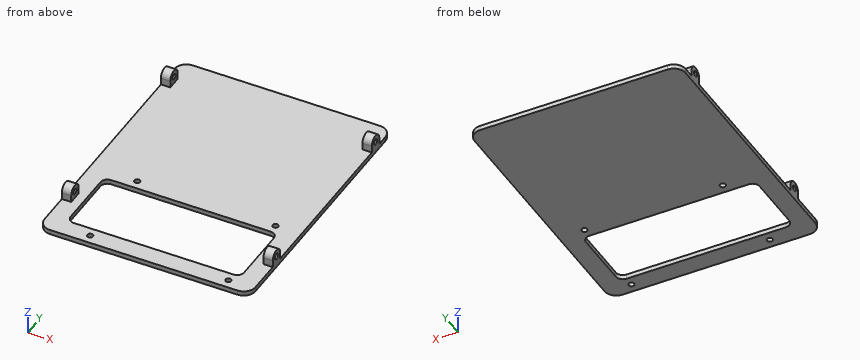
```python
from build123d import *

# Parameters (mm, degrees)
SKETCH1_R                        = 1.524
SCREW_HOLES_DEPTH                = 5.08
SCREW_HOLES_2_DEPTH              = 5.08
SKETCH2_W                        = 2.54
SKETCH2_H                        = 146.05
MAIN_EXTRUDE_DEPTH               = 114.3
FILLET1_R                        = 6.35
SKETCH3_R                        = 1.524
COMPONENT_MOUNT_HOLES_DEPTH      = 8.62
COMPONENT_MOUNT_HOLES_DEPTH_BACK = 3.54
SKETCH4_W                        = 93.98
SKETCH4_H                        = 38.1
WEIGHT_REDUCTION_DEPTH           = 8.62
WEIGHT_REDUCTION_DEPTH_BACK      = 3.54
FILLET2_R                        = 3.81


with BuildPart() as part:
    # Sketch1 → Screw holes (new body)
    with BuildSketch(Plane(origin=(0, 0, 0), x_dir=(0, 0, -1), z_dir=(1, 0, 0))):
        with BuildLine():
            Line((0, 46.99), (3.81, 46.99))
            Line((3.81, 46.99), (3.81, 54.61))
            Line((3.81, 54.61), (0, 54.61))
            ThreePointArc((0, 54.61), (-3.81, 50.8), (0, 46.99))
        make_face()
        with Locations((0, 50.8)):
            Circle(SKETCH1_R, mode=Mode.SUBTRACT)
    screw_holes = extrude(amount=SCREW_HOLES_DEPTH)



with BuildPart() as body_2:
    # Sketch1 → Screw holes 2 (new body)
    with BuildSketch(Plane(origin=(0, 0, 0), x_dir=(0, 0, -1), z_dir=(1, 0, 0))):
        with BuildLine():
            Line((3.81, -54.61), (0, -54.61))
            ThreePointArc((0, -54.61), (-3.81, -50.8), (0, -46.99))
            Line((0, -46.99), (3.81, -46.99))
            Line((3.81, -46.99), (3.81, -54.61))
        make_face()
        with Locations((0, -50.8)):
            Circle(SKETCH1_R, mode=Mode.SUBTRACT)
    screw_holes_2 = extrude(amount=SCREW_HOLES_2_DEPTH)


with BuildPart() as part_1:
    add(part.part)

    add(body_2.part)  # Main extrude merges body 2
    # Sketch2 → Main extrude (add)
    with BuildSketch(Plane.ZY):
        with Locations((-5.08, -5.715)):
            Rectangle(SKETCH2_W, SKETCH2_H)
    extrude(amount=-MAIN_EXTRUDE_DEPTH)

    # Screw holes 2 2: Screw holes, Screw holes 2 across plane
    add(screw_holes.mirror(Plane.ZY.offset(-57.15)))
    add(screw_holes_2.mirror(Plane.ZY.offset(-57.15)))

    # Fillet1
    fillet1_edges = [part_1.edges().sort_by_distance(p)[0] for p in [
        (114.3, -78.74, -5.08),
        (114.3, 67.31, -5.08),
        (0, 67.31, -5.08),
        (0, -78.74, -5.08),
    ]]
    fillet(fillet1_edges, radius=FILLET1_R)

    # Sketch3 → Component mount holes (cut, two sides)
    with BuildSketch(Plane.XY.offset(-3.81)) as component_mount_holes_sk:
        with Locations((25.4, -25.4)):
            Circle(SKETCH3_R)
        with Locations((100.33, -25.4)):
            Circle(SKETCH3_R)
        with Locations((100.33, -73.66)):
            Circle(SKETCH3_R)
        with Locations((25.4, -73.66)):
            Circle(SKETCH3_R)
    extrude(amount=COMPONENT_MOUNT_HOLES_DEPTH, mode=Mode.SUBTRACT)
    extrude(component_mount_holes_sk.sketch, amount=-COMPONENT_MOUNT_HOLES_DEPTH_BACK, mode=Mode.SUBTRACT)

    # Sketch4 → Weight reduction (cut, two sides)
    with BuildSketch(Plane.XY.offset(-3.81)) as weight_reduction_sk:
        with Locations((57.15, -49.53)):
            Rectangle(SKETCH4_W, SKETCH4_H)
    extrude(amount=WEIGHT_REDUCTION_DEPTH, mode=Mode.SUBTRACT)
    extrude(weight_reduction_sk.sketch, amount=-WEIGHT_REDUCTION_DEPTH_BACK, mode=Mode.SUBTRACT)

    # Fillet2
    fillet2_edges = [part_1.edges().sort_by_distance(p)[0] for p in [
        (10.16, -68.58, -5.08),
        (10.16, -30.48, -5.08),
        (104.14, -30.48, -5.08),
        (104.14, -68.58, -5.08),
    ]]
    fillet(fillet2_edges, radius=FILLET2_R)


solid = part_1.part
```
Input: part model. Units: mm. Frame: model coordinates. Coordinates: 2 decimals unless noted, no trailing zeros. Write each loop counter-clockwise with the first axis right and the second up, starting at its lowest first coordinate (ties: lowest second). Pieces come first, ordered by that corner, then holes. Notation, with made-up numbers: (-15.5, 47) - (34.5, 47) arc R22 ccw to (34.5, 80) - close; hole circle Ø5 at (-11.75, -11.5). An arc over 180 degrees is marked (long way). Put each result on its own line as item: value. Start each with the question number.
1) Cut plane D-D (y = 50.8). Return the cut outline in (x, z).
2) Cut plane A-A (y = -56.5). Return the cut outline in (x, z), plus the area to 3 significant figures.
3) Contact query for flat-ended pins moving along their axis: pin 1 (1.1 mm diameter, centred on x = 112, z = -2, fed in from -Y); pin 2 (5 mm diameter, centred on x = 25.4, y = -73.66, fed in from +Z); pin 3 (2.5 mm diameter, centred on y = -50.8, z = 0, fed in from -X); pin 4 (3 mm diameter, centred on x = 112, z = -2, fed in from +Y). Output: stop coordinate, or through.
4) Cut plane B-B (x = 25.4). Return the cut outline in (y, z).
5) Ray query, L1, parallel to Y at x = 100.33, z = -5.5; L2, parallel to X at y = -56.5, z = -4.5; L3, parallel to Z at x = 62.5, y = -7.5. Return the intervals inside material, ascending.
6) Cut plane C-C (y = -25.4). Return the cut outline in (x, z).
Resolved:
1. outline: (0, -6.35) - (114.3, -6.35) - (114.3, -1.52) - (109.22, -1.52) - (109.22, -3.81) - (5.08, -3.81) - (5.08, -1.52) - (0, -1.52) - close; (0, 1.52) - (5.08, 1.52) - (5.08, 3.81) - (0, 3.81) - close; (109.22, 1.52) - (114.3, 1.52) - (114.3, 3.81) - (109.22, 3.81) - close
2. outline: (0, -6.35) - (10.16, -6.35) - (10.16, -3.81) - (0, -3.81) - close; (104.14, -6.35) - (114.3, -6.35) - (114.3, -3.81) - (104.14, -3.81) - close
2. area: 51.6 mm2
3. pin 1: stops at y = -54.61
3. pin 2: stops at z = -3.81
3. pin 3: passes through
3. pin 4: stops at y = 54.61
4. outline: (-78.74, -6.35) - (-75.18, -6.35) - (-75.18, -3.81) - (-78.74, -3.81) - close; (-72.14, -6.35) - (-68.58, -6.35) - (-68.58, -3.81) - (-72.14, -3.81) - close; (-30.48, -6.35) - (-26.92, -6.35) - (-26.92, -3.81) - (-30.48, -3.81) - close; (-23.88, -6.35) - (67.31, -6.35) - (67.31, -3.81) - (-23.88, -3.81) - close
5. L1: y = -78.74 to -75.18, -72.14 to -68.58, -30.48 to -26.92, -23.88 to 67.31
5. L2: x = 0 to 10.16, 104.14 to 114.3
5. L3: z = -6.35 to -3.81
6. outline: (0, -6.35) - (23.88, -6.35) - (23.88, -3.81) - (0, -3.81) - close; (26.92, -6.35) - (98.81, -6.35) - (98.81, -3.81) - (26.92, -3.81) - close; (101.85, -6.35) - (114.3, -6.35) - (114.3, -3.81) - (101.85, -3.81) - close
